CAD build for the part. Positions are in the model's coordinates, mm. A direction names the side the tool comes from. Give positions to 0.01 mm unless a question says otherwise; leave off trailing zeros. Write each loop counter-clockwise with the first axis right and the second up, starting at its lowest first coordinate (ties: lowest second). Pieces come first, ordered by that corner, then holes. Notation, with made-up numbers: (39, -31) -> (49, -31) arc R24 ccw to (49, -17) -> close; hole circle Ø3 at (-28.5, 54.5). An arc over 180 degrees is marked (long way). Answer as a JSON object with one key per item and string values.
```python
from build123d import *

# Parameters (mm, degrees)
SKETCH1_W           = 50
SKETCH1_H           = 60
BOSS_EXTRUDE1_DEPTH = 5
SKETCH2_W           = 10
SKETCH2_H           = 60
BOSS_EXTRUDE2_DEPTH = 45
SKETCH3_R           = 2.5
CUT_EXTRUDE1_DEPTH  = 60.581876439
CUT_EXTRUDE2_REACH  = 67.574
SKETCH5_R           = 2.5
FILLET1_R           = 3


with BuildPart() as part:
    # Sketch1 → Boss-Extrude1 (new body)
    with BuildSketch(Plane(origin=(0, 0, 0), x_dir=(1, 0, 0), z_dir=(0, 1, 0))):
        Rectangle(SKETCH1_W, SKETCH1_H)
    extrude(amount=BOSS_EXTRUDE1_DEPTH)

    # Sketch2 → Boss-Extrude2 (add)
    with BuildSketch(Plane(origin=(0, 5, 0), x_dir=(1, 0, 0), z_dir=(0, 1, 0))):
        Rectangle(SKETCH2_W, SKETCH2_H)
    extrude(amount=BOSS_EXTRUDE2_DEPTH)

    # Sketch3 → Cut-Extrude1 (cut, through all)
    with BuildSketch(Plane(origin=(0, 5, 0), x_dir=(1, 0, 0), z_dir=(0, 1, 0))):
        with Locations(Location((-15.028328695, 0, 0), (0, 0, 270))):
            Circle(SKETCH3_R)
        with Locations(Location((15.028328695, 0, 0), (0, 0, 270))):
            Circle(SKETCH3_R)
    extrude(amount=-CUT_EXTRUDE1_DEPTH, mode=Mode.SUBTRACT)

    # Sketch5 → Cut-Extrude2 (cut, up to next)
    with BuildSketch(Plane.ZY.offset(5), mode=Mode.PRIVATE) as cut_extrude2_sk1:
        with Locations((-19, 27.5)):
            Circle(SKETCH5_R)
    cut_extrude2_tool1 = extrude(cut_extrude2_sk1.sketch, amount=-CUT_EXTRUDE2_REACH, mode=Mode.PRIVATE) & part.part
    # Sketch5 → Cut-Extrude2 (cut, up to next)
    with BuildSketch(Plane.ZY.offset(5), mode=Mode.PRIVATE) as cut_extrude2_sk2:
        with Locations((19, 27.5)):
            Circle(SKETCH5_R)
    cut_extrude2_tool2 = extrude(cut_extrude2_sk2.sketch, amount=-CUT_EXTRUDE2_REACH, mode=Mode.PRIVATE) & part.part
    add(cut_extrude2_tool1.solids().sort_by_distance((-5, 27.5, -19))[0], mode=Mode.SUBTRACT)
    add(cut_extrude2_tool2.solids().sort_by_distance((-5, 27.5, 19))[0], mode=Mode.SUBTRACT)

    # Fillet1
    fillet1_edges = [part.edges().sort_by_distance(p)[0] for p in [
        (5, 5, 0),
        (-5, 5, 0),
    ]]
    fillet(fillet1_edges, radius=FILLET1_R)


solid = part.part
```
1) Slice it at D-D (y = 42). List the corners of the cut face in (x, z), then the cut area to 3 significant figures.
Model answer:
{"outline": "(-5, -30) -> (5, -30) -> (5, 30) -> (-5, 30) -> close", "area": "600 mm2"}
2) Slice it at A-A (z = 0). List the corners of the cut face in (x, y), then the cut area to 3 significant figures.
Model answer:
{"outline": "(-25, 0) -> (-17.53, 0) -> (-17.53, 5) -> (-25, 5) -> close; (-12.53, 0) -> (12.53, 0) -> (12.53, 5) -> (8, 5) arc R3 cw to (5, 8) -> (5, 50) -> (-5, 50) -> (-5, 8) arc R3 cw to (-8, 5) -> (-12.53, 5) -> close; (17.53, 0) -> (25, 0) -> (25, 5) -> (17.53, 5) -> close", "area": "654 mm2"}
3) 3-axis set-ups, long thin cutter, end or side, ignore diameter. For faces 4 (the flat face through (-19, 5, 0)), 5 (the flat face through (0, 50, 0)), 6 (the flat face through (5, 29, 0)): which of +Z, -Z, +X, -X, +Y, -Y reach the whole face in a straight line?
Model answer:
{"face 4": "+Z, -Z, -X, +Y", "face 5": "+Z, -Z, +X, -X, +Y", "face 6": "+Z, -Z, +X, +Y"}
4) Slice it at B-B (z = -19). List the corners of the cut face in (x, y), then the cut area to 3 significant figures.
Model answer:
{"outline": "(-25, 0) -> (25, 0) -> (25, 5) -> (8, 5) arc R3 cw to (5, 8) -> (5, 25) -> (-5, 25) -> (-5, 8) arc R3 cw to (-8, 5) -> (-25, 5) -> close; (-5, 30) -> (5, 30) -> (5, 50) -> (-5, 50) -> close", "area": "654 mm2"}
5) Pin check, flat tips, straight feed: pin 1 (12 mm diameter, centred on x = -4.5, z = 18.5, fed in from -Y); pin 2 (3 mm diameter, centred on y = 31.5, z = -4, fed in from +X); pin 3 (4 mm diameter, centred on y = 27.5, z = 19, fed in from +X); pin 4 (12.5 mm diameter, centred on y = 31, z = 5, fed in from -X). Stop position of each tip, or through.
Model answer:
{"pin 1": "stops at y = 0", "pin 2": "stops at x = 5", "pin 3": "passes through", "pin 4": "stops at x = -5"}
6) Mould opens along X. For faces 1 (the cylindrical face through (-12.55, 2.54, -0.33)), 2 (the flat face through (0, 19, -30)), 3 (the flat face through (-5, 29, 0)) say: released by +X, released by -X, zero draft, split by the parting line, or undercut.
Model answer:
{"face 1": "undercut", "face 2": "zero draft", "face 3": "released by -X"}
7) Slice it at C-C (x = 14). List the corners of the cut face in (y, z), then the cut area to 3 significant figures.
Model answer:
{"outline": "(0, -30) -> (5, -30) -> (5, -2.28) -> (0, -2.28) -> close; (0, 2.28) -> (5, 2.28) -> (5, 30) -> (0, 30) -> close", "area": "277 mm2"}
8) Wall check: probe 1 along X at (y, z) = (2, 0); probe 2 along Z at (x, y) = (0, 27); probe 3 along Y at (x, z) = (-2.5, -19). Give the ranges that are in metal, low to high.
Model answer:
{"probe 1": "x = -25 to -17.53, -12.53 to 12.53, 17.53 to 25", "probe 2": "z = -30 to -21.45, -16.55 to 16.55, 21.45 to 30", "probe 3": "y = 0 to 25, 30 to 50"}
